Could you check a few things on this model? Use its own coordinates, in mm. A direction names the side the tool comes from. Coordinates: 2 decimals unless noted, no trailing zeros. Order: outer loops, then holes, each group sorted by start corner. A loop starts at its lowest first (then second) coordinate and runs counter-clockwise, first axis right, second up. Notation, with made-up numbers: (89, 67.25) - (100, 67.25) arc R30 ccw to (100, 104.25) - close; hole circle Ø8 at (24.5, 43). An arc over 180 degrees is marked (long way). Answer as CSV lines item,"result". Start each with the question number.
1. Thinking about a two-plate mould opening in X: for faces 6 (the face through (56.42, -0.04, 39.94)), 7 (the face through (-67.327, 0.044, 44.537)), 8 (the face through (-24, 0, 57.002)), which applies, released by +X, released by -X, zero draft, split by the parting line, or undercut?
2. I want a section at B-B, the plane y = -0.5. List the corners of the cut face in (x, z) for me (3 decimals), and give its area (3 significant figures).
3. I want a section at D-D, the plane x = 29.5. List the corners of the cut face in (y, z) for me (3 decimals).
4. For pin 1 (2 mm diameter, centred on y = -0.5, z = 40, fed in from +X); pin 2 (3 mm diameter, centred on x = 16, y = -1, fed in from -Z); pin 3 (3 mm diameter, centred on x = -36, y = 0.5, fed in from +Z), each with a flat end and sliding along its axis, tell me the tip position at first contact or that it passes through.
5. I want a section at C-C, the plane z = 38.1. List the corners of the cut face in (x, y) for me (3 decimals).
6. For faces 1 (the face through (-66, 0, 15.24)), 2 (the face through (-79.293, 0, -27)), 3 (the face through (-25, 0, -57.002)), 4 (the face through (22, 0, 18.28)), 5 (the face through (30.21, -0.04, 51.48)), which set-ups out of +Z, -Z, +X, -X, +Y, -Y let a thin tool reach every point of the face, with its end or its side?
7. I want a section at A-A, the plane x = -15.5. List the corners of the cut face in (y, z) for me (3 decimals), and give its area (3 significant figures).
8. I need wall thicknesses on probe 1 along X at (y, z) = (-0.5, -41); probe 2 along Z at (x, y) = (-67, 2); probe 3 along X at (y, z) = (-1.5, 39.5). Which ranges of each line are inside material? Lowest first, please.
from build123d import *

# Parameters (mm, degrees)
F0_R     = 9.525
F0_R_2   = 7.91296
F1_DEPTH = 3.175


with BuildPart() as f1:
    # F0 (on Front) → F1 (new body, symmetric)
    with BuildSketch(Plane.XZ):
        with BuildLine():
            ThreePointArc((-57.934586, 57.001762), (-60.306483, 57.15), (-62.67838, 57.001762))
            Line((-62.67838, 57.001762), (-57.934586, 57.001762))
        make_face()
        with BuildLine():
            Line((-57.934586, 57.001762), (-62.67838, 57.001762))
            ThreePointArc((-62.67838, 57.001762), (-74.064603, 51.276367), (-79.29303, 39.653556))
            Line((-79.29303, 39.653556), (-79.29303, 15.24))
            Line((-79.29303, 15.24), (-51.752072, 15.24))
            ThreePointArc((-51.752072, 15.24), (-26.806955, 25.649029), (0, 29.112254))
            ThreePointArc((0, 29.112254), (4.725363, 24.672997), (5.803779, 18.279791))
            Line((5.803779, 18.279791), (38.5414, 18.279791))
            Line((38.5414, 18.279791), (38.5414, 0))
            Line((38.5414, 0), (38.5414, -18.279791))
            Line((38.5414, -18.279791), (5.803779, -18.279791))
            ThreePointArc((5.803779, -18.279791), (4.725363, -24.672997), (0, -29.112254))
            ThreePointArc((0, -29.112254), (-26.806955, -25.649029), (-51.752072, -15.24))
            Line((-51.752072, -15.24), (-79.29303, -15.24))
            Line((-79.29303, -15.24), (-79.29303, -39.653556))
            ThreePointArc((-79.29303, -39.653556), (-74.064603, -51.276367), (-62.67838, -57.001762))
            Line((-62.67838, -57.001762), (-57.934586, -57.001762))
            Line((-57.934586, -57.001762), (9.60697, -57.001762))
            Line((9.60697, -57.001762), (50.24697, -46.112307))
            Line((50.24697, -46.112307), (62.4174, -33.941876))
            Line((62.4174, -33.941876), (62.4174, -5.23346))
            Line((62.4174, -5.23346), (62.4174, 5.23346))
            Line((62.4174, 5.23346), (62.4174, 33.941876))
            Line((62.4174, 33.941876), (50.24697, 46.112307))
            Line((50.24697, 46.112307), (9.60697, 57.001762))
            Line((9.60697, 57.001762), (-57.934586, 57.001762))
        make_face()
        with Locations((-60.306483, -38.1)):
            Circle(F0_R, mode=Mode.SUBTRACT)
        with Locations((28.593517, -35.27448)):
            Circle(F0_R_2, mode=Mode.SUBTRACT)
        with Locations((-60.306483, 38.1)):
            Circle(F0_R, mode=Mode.SUBTRACT)
        with Locations((28.593517, 35.27448)):
            Circle(F0_R_2, mode=Mode.SUBTRACT)
        with BuildLine():
            ThreePointArc((-62.67838, -57.001762), (-60.306483, -57.15), (-57.934586, -57.001762))
            Line((-57.934586, -57.001762), (-62.67838, -57.001762))
        make_face()
    extrude(amount=F1_DEPTH, both=True)


solid = f1.part
Solved:
1,face 6,"released by +X"
1,face 7,"undercut"
1,face 8,"zero draft"
2,outline,"(-79.293, -39.654) arc R19.05 ccw to (-62.678, -57.002) arc R19.05 ccw to (-57.935, -57.002) - (9.607, -57.002) - (50.247, -46.112) - (62.417, -33.942) - (62.417, 33.942) - (50.247, 46.112) - (9.607, 57.002) - (-57.935, 57.002) arc R19.05 ccw to (-62.678, 57.002) arc R19.05 ccw to (-79.293, 39.654) - (-79.293, 15.24) - (-51.752, 15.24) arc R101.6 cw to (0, 29.112) arc R10.16 cw to (5.804, 18.28) - (38.541, 18.28) - (38.541, -18.28) - (5.804, -18.28) arc R10.16 cw to (0, -29.112) arc R101.6 cw to (-51.752, -15.24) - (-79.293, -15.24) - close; hole circle Ø19.05 at (-60.306, -38.1); hole circle Ø19.05 at (-60.306, 38.1); hole circle Ø15.826 at (28.594, -35.274); hole circle Ø15.826 at (28.594, 35.274)"
2,area,"9,290 mm2"
3,outline,"(-3.175, -51.671) - (3.175, -51.671) - (3.175, -43.135) - (-3.175, -43.135) - close; (-3.175, -27.414) - (3.175, -27.414) - (3.175, -18.28) - (-3.175, -18.28) - close; (-3.175, 18.28) - (3.175, 18.28) - (3.175, 27.414) - (-3.175, 27.414) - close; (-3.175, 43.135) - (3.175, 43.135) - (3.175, 51.671) - (-3.175, 51.671) - close"
4,pin 1,"stops at x = 57.36"
4,pin 2,"stops at z = -55.69"
4,pin 3,"stops at z = 57"
5,outline,"(-79.293, -3.175) - (-69.831, -3.175) - (-69.831, 3.175) - (-79.293, 3.175) - close; (-50.781, -3.175) - (21.202, -3.175) - (21.202, 3.175) - (-50.781, 3.175) - close; (35.985, -3.175) - (58.259, -3.175) - (58.259, 3.175) - (35.985, 3.175) - close"
6,face 1,"-X, +Y, -Y"
6,face 2,"+Z, -Z, -X, +Y, -Y"
6,face 3,"-Z, +X, +Y, -Y"
6,face 4,"+Y, -Y"
6,face 5,"+Z, +X, +Y, -Y"
7,outline,"(-3.175, -57.002) - (3.175, -57.002) - (3.175, -28) - (-3.175, -28) - close; (-3.175, 28) - (3.175, 28) - (3.175, 57.002) - (-3.175, 57.002) - close"
7,area,"368 mm2"
8,probe 1,"x = -79.13 to -69.38, -51.23 to 23.13, 34.06 to 55.36"
8,probe 2,"z = -55.94 to -44.88, -31.32 to -15.24, 15.24 to 31.32, 44.88 to 55.94"
8,probe 3,"x = -79.29 to -69.73, -50.88 to 21.9, 35.28 to 56.86"
